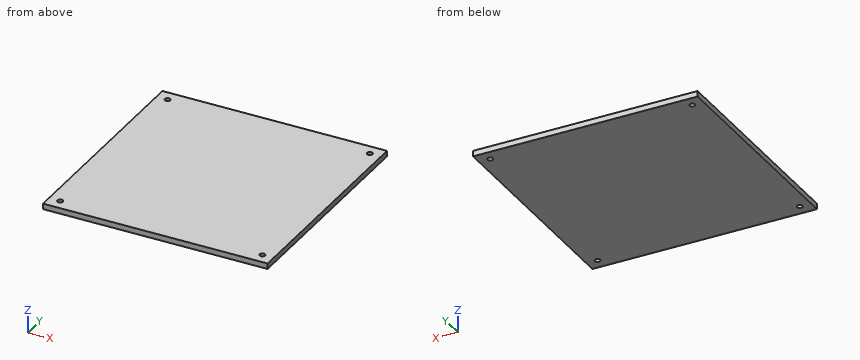
Autodesk Inventor part; units mm, degrees
ref_plane "YZ Plane" through (0, 0, 0) normal (1, 0, 0) x (0, 1, 0)
ref_plane "XZ Plane" through (0, 0, 0) normal (0, 1, 0) x (-1, 0, 0)
ref_plane "XY Plane" through (0, 0, 0) normal (0, 0, 1) x (1, 0, 0)
sketch "Sketch1" plane through (0, 0, 0) normal (0, 0, 1) x (1, 0, 0)
  line L0 (-63.5, 63.5) -> (63.5, 63.5)
  line L1 (63.5, 63.5) -> (63.5, -63.5)
  line L2 (63.5, -63.5) -> (-63.5, -63.5)
  line L3 (-63.5, -63.5) -> (-63.5, 63.5)
  circle A0 centre (-57.15, 57.15) radius 1.524
  circle A1 centre (57.15, 57.15) radius 1.524
  line L4 (63.5, 0) -> (-63.5, 0)
  circle A2 centre (-57.15, -57.15) radius 1.524
  circle A3 centre (57.15, -57.15) radius 1.524
  point P0 (0, 0)
  point P1 (0, 63.5)
  dimension "d0" = 127
  dimension "d1" = 127
  dimension "d2" = 127
  dimension "d3" = 3.048
  dimension "d4" = 3.048
  dimension "d5" = 6.35
  dimension "d6" = 6.35
  dimension "d7" = 6.35
  dimension "d8" = 6.35
extrude "Extrusion1" add sketch "Sketch1" along normal blind 3.175
properties part number "hank - base 1"
For this review, take the finished solid that the model builds, in its own axes (mm). Coordinates: 2 decimals unless noted, no trailing zeros. Order: outer loops, then holes, each group sorted by start corner. A loop starts at its lowest first (then second) coordinate and runs counter-clockwise, first axis right, second up. Notation, with made-up numbers: (43.5, 11.5) -> (100.5, 11.5) arc R27 cw to (100.5, 28.5) -> close; hole circle Ø7 at (58, -23.75). An arc over 180 degrees is marked (long way). Return JSON: item names as keys, results as strings.
1. For pin 1 Ø2.5 at (x, y) = (-57.15, -57.15) entering from -Z, flat-tipped, find the tip position at first contact; note if it passes through.
Answer block:
{"pin 1": "through"}
2. We need section A-A on x = 57.15. Write out the cut boundary in (y, z) (3 decimals), and give its area (3 significant figures).
Answer block:
{"outline": "(-63.5, 0) -> (-58.674, 0) -> (-58.674, 3.175) -> (-63.5, 3.175) -> close; (-55.626, 0) -> (55.626, 0) -> (55.626, 3.175) -> (-55.626, 3.175) -> close; (58.674, 0) -> (63.5, 0) -> (63.5, 3.175) -> (58.674, 3.175) -> close", "area": "384 mm²"}
3. For line 1 (Y direction, x = -57.15, z = 2.1); line 2 (Y direction, x = -57.5, z = 2.45), list the stretches that pass through material, from the lowest coordinate up. Write a range as from..to.
Answer block:
{"line 1": "-63.5..-58.67, -55.63..55.63, 58.67..63.5", "line 2": "-63.5..-58.63, -55.67..55.67, 58.63..63.5"}
